Design review of the part shown in the three views and the two pictorial views. Dimensions are in mm from the part's minimum x, y and z. A direction names the side the tool comes from. Round coordinates to 2 decimals unless told otherwise and drop trailing zeros. Loops run counter-clockwise (first coordinate to the right, second up) from the corner with the lowest first, then second, coordinate; pieces in that order, holes last.
1. Tool access review of the marked faces 1 and 2: name each direction out of +Z, -Z, +X, -X, +Y, -Y from which nothing blocks a thin tool from reaching the whole face with its end or side.
2. Consider section D-D on x = 6. State the section outline as (y, z) points.
3. To check wall thickness, follow line 1 along X through (y, z) = (1.7, 7.5); line 2 along X through (y, z) = (1.05, 7.5); line 3 along Z through (x, y) = (10, 0.9). State the ranges of each line that lie inside material, in increasing order.
4. Consider section A-A on z = 7.5. State the section outline as (x, y) points.
5. Clearance check with flat-ended pins moving along their axes: pin 1 Ø5 at (x, z) = (8.5, 8) entering from +Y; pin 2 Ø2.5 at (x, z) = (50, 7.5) entering from -Y. State where each tip first meets the part, or that it passes through.
6. Consider section C-C on x = 51. State the section outline as (y, z) points, then the cut area to 3 significant figures.
7. Consider section B-B on y = 1.2. State the section outline as (x, z) points.
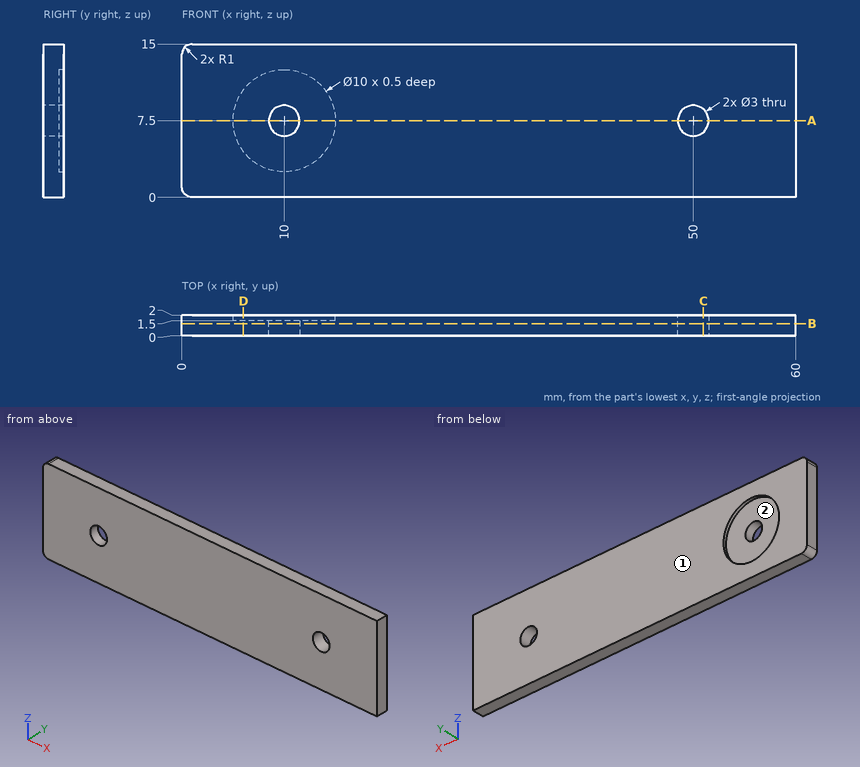
Resolved:
1. face 1: +Z, -Z, +X, -X, +Y
1. face 2: +Y
2. outline: (0, 0) - (2, 0) - (2, 4.5) - (1.5, 4.5) - (1.5, 10.5) - (2, 10.5) - (2, 15) - (0, 15) - close
3. line 1: x = 0 to 5, 15 to 48.5, 51.5 to 60
3. line 2: x = 0 to 8.5, 11.5 to 48.5, 51.5 to 60
3. line 3: z = 0 to 6, 9 to 15
4. outline: (0, 0) - (8.5, 0) - (8.5, 1.5) - (5, 1.5) - (5, 2) - (0, 2) - close; (11.5, 0) - (48.5, 0) - (48.5, 2) - (15, 2) - (15, 1.5) - (11.5, 1.5) - close; (51.5, 0) - (60, 0) - (60, 2) - (51.5, 2) - close
5. pin 1: stops at y = 1.5
5. pin 2: passes through
6. outline: (0, 0) - (2, 0) - (2, 6.38) - (0, 6.38) - close; (0, 8.62) - (2, 8.62) - (2, 15) - (0, 15) - close
6. area: 25.5 mm2
7. outline: (0, 1) arc R1 ccw to (1, 0) - (60, 0) - (60, 15) - (1, 15) arc R1 ccw to (0, 14) - close; hole circle Ø3 at (10, 7.5); hole circle Ø3 at (50, 7.5)
